Part model, mm, in its own coordinate system. A direction names the side the tool comes from. Round coordinates to 2 decimals unless told otherwise and drop trailing zeros. Order: outer loops, then holes, each group sorted by start corner. A loop starts at its lowest first (then second) coordinate and runs counter-clockwise, first axis right, second up. Notation, with made-up numbers: (27.5, -0.5) - (31.5, -0.5) arc R22 ccw to (31.5, 8.5) - close; hole circle Ø6 at (-25.5, 56). An arc over 180 degrees is marked (long way). Answer as a JSON object with one key per item and string values.
```python
from build123d import *

# Parameters (mm, degrees)
BOSS_EXTRUDE1_DEPTH = 19.05
FILLET1_R           = 2.54


with BuildPart() as part:
    # Sketch1 → Boss-Extrude1 (new body, symmetric)
    with BuildSketch(Plane(origin=(0, 0, 0), x_dir=(1, 0, 0), z_dir=(0, 1, 0))):
        with BuildLine():
            Line((-19.446875, 31.353125), (-19.446875, 11.90625))
            ThreePointArc((-19.446875, 11.90625), (-13.751017173, 25.657267198), (3.5e-08, 31.353125))
            Line((3.5e-08, 31.353125), (-19.446875, 31.353125))
        make_face()
        with BuildLine():
            Line((19.446875, 0), (19.446875, 11.90625))
            ThreePointArc((19.446875, 11.90625), (0, 31.353125), (-19.446875, 11.90625))
            Line((-19.446875, 11.90625), (-19.446875, 0))
            ThreePointArc((-19.446875, 0), (0, -19.446875), (19.446875, 0))
        make_face()
        with BuildLine():
            ThreePointArc((13.096875, 11.90625), (0, 25.003125), (-13.096875, 11.90625))
            Line((-13.096875, 11.90625), (-13.096875, 0))
            ThreePointArc((-13.096875, 0), (0, -13.096875), (13.096875, 0))
            Line((13.096875, 0), (13.096875, 11.90625))
        make_face(mode=Mode.SUBTRACT)
        with BuildLine():
            Line((19.446875, 31.353125), (3.5e-08, 31.353125))
            ThreePointArc((3.5e-08, 31.353125), (13.751017198, 25.657267173), (19.446875, 11.90625))
            Line((19.446875, 11.90625), (19.446875, 31.353125))
        make_face()
    extrude(amount=BOSS_EXTRUDE1_DEPTH, both=True)

    # Sketch2 → Cut-Revolve1 (revolve, cut)
    with BuildSketch(Plane(origin=(0, 7.9375, 0), x_dir=(1, 0, 0), z_dir=(0, 1, 0))):
        Polygon((-2.06375, 31.353125), (-2.06375, 26.433924349), (-4.445, 25.003125), (-4.445, 0), (-5.55625, 0), (-5.55625, -19.446875), (-4.445, -19.446875), (0, -19.446875), (0, 31.353125), align=None)
    cut_revolve1 = revolve(axis=Axis((0, 7.9375, -28.179060189), (0, 0, 1)), mode=Mode.SUBTRACT)

    # Mirror1: Cut-Revolve1 across plane
    add(cut_revolve1.mirror(Plane.ZX), mode=Mode.SUBTRACT)

    # Fillet1
    fillet1_edges = [part.edges().sort_by_distance(p)[0] for p in [
        (-13.096875, -19.05, -5.953125),
        (0, -19.05, 13.096875),
        (13.096875, -19.05, -5.953125),
        (0, -19.05, -25.003125),
        (0, 19.05, 19.446875),
        (19.446875, -19.05, -15.6765625),
        (0, -19.05, 19.446875),
        (-19.446875, -19.05, -15.6765625),
        (19.446875, 19.05, -15.6765625),
        (0, 19.05, -25.003125),
        (13.096875, 19.05, -5.953125),
        (0, 19.05, 13.096875),
        (-13.096875, 19.05, -5.953125),
        (-19.446875, 19.05, -15.6765625),
    ]]
    fillet(fillet1_edges, radius=FILLET1_R)


solid = part.part
```
Item 1: Two-plate mould, pull along X, no slides. Class faces 5 (the flat face through (-19.447, 0, -16)), 6 (the cylindrical face through (-2.56, -12.87, 15.71)), 7 (the flat face through (0, 0, -31.353)): pulls with the +X half, pulls with the -X half, needs draft (parallel to the pull), parting line crosses it, or undercut.
Taken from the geometry:
{"face 5": "pulls with the -X half", "face 6": "undercut", "face 7": "needs draft"}
Item 2: Tool access for faces 1 (the cylindrical face through (4.444, -7.84, -24.695)), 2 (the cylindrical face through (-0.288, 0.231, 13.094)), 3 (the cylindrical face through (-18.68, 18.33, -15.46)), 4 (the cylindrical face through (13.821, -18.286, -6.036)): list every direction of +Z, -Z, +X, -X, +Y, -Y with a clear straight run to the whole face (end or side of a thin tool).
Taken from the geometry:
{"face 1": "+Z", "face 2": "+Y, -Y", "face 3": "+Z, -Z, -X, +Y", "face 4": "-Y"}
Item 3: Drop flat-ended pins along their axis: P1, Ø2, axis at y = 1.5, z = 5, coming from the -X side; P2, Ø10, axis at x = 0, y = 7.94, coming from the +Z side; P3, Ø1.5, axis at x = -13, z = -14.5, coming from the -Y side. Give the stop position or say it passes through.
Taken from the geometry:
{"P1": "x = -19.03", "P2": "z = -24.01", "P3": "y = -18.46"}
Item 4: Probe L1, parallel to Y at x = 0, z = 16; L2, parallel to Y at x = 0, z = -27.9; L3, parallel to X at y = 15, z = -9.5. List the from-to ranges inside material, lowest first. Write a range as from..to.
Taken from the geometry:
{"L1": "-19.05..-13.49, -2.38..2.38, 13.49..19.05", "L2": "-19.05..-10, -5.87..5.87, 10..19.05", "L3": "-19.45..-13.1, 13.1..19.45"}
Item 5: Cut at A-A (z = -10.5). Write the cut outline in (x, y), plus the area to 3 significant figures.
Taken from the geometry:
{"outline": "(-19.45, -16.51) arc R2.54 ccw to (-16.91, -19.05) - (-15.64, -19.05) arc R2.54 ccw to (-13.1, -16.51) - (-13.1, 16.51) arc R2.54 ccw to (-15.64, 19.05) - (-16.91, 19.05) arc R2.54 ccw to (-19.45, 16.51) - close; (13.1, -16.51) arc R2.54 ccw to (15.64, -19.05) - (16.91, -19.05) arc R2.54 ccw to (19.45, -16.51) - (19.45, 16.51) arc R2.54 ccw to (16.91, 19.05) - (15.64, 19.05) arc R2.54 ccw to (13.1, 16.51) - close", "area": "473 mm2"}
Item 6: Cut at B-B (y = -0.5). Write the cut outline in (x, z), plus the area to 3 significant figures.
Taken from the geometry:
{"outline": "(-19.45, -31.35) - (19.45, -31.35) - (19.45, 0) arc R19.45 ccw to (-19.45, 0) - close; hole (-13.1, -11.91) arc R13.1 ccw to (13.1, -11.91) - (13.1, 0) arc R13.1 ccw to (-13.1, 0) - close", "area": "963 mm2"}
